from build123d import *

# Parameters (mm, degrees)
SKETCH1_W           = 190
SKETCH1_H           = 120
SKETCH1_R           = 6
SKETCH1_R_2         = 10
SKETCH1_R_3         = 2
BOSS_EXTRUDE1_DEPTH = 5


with BuildPart() as part:
    # Sketch1 → Boss-Extrude1 (new body)
    with BuildSketch(Plane.XY):
        Rectangle(SKETCH1_W, SKETCH1_H)
        with Locations((-75, 30)):
            Circle(SKETCH1_R, mode=Mode.SUBTRACT)
        with Locations((75, 30)):
            Circle(SKETCH1_R, mode=Mode.SUBTRACT)
        with Locations((75, -30)):
            Circle(SKETCH1_R, mode=Mode.SUBTRACT)
        with Locations((-75, -30)):
            Circle(SKETCH1_R, mode=Mode.SUBTRACT)
        Circle(SKETCH1_R_2, mode=Mode.SUBTRACT)
        with Locations((0, 16)):
            Circle(SKETCH1_R_3, mode=Mode.SUBTRACT)
        with Locations((13.856406461, 8)):
            Circle(SKETCH1_R_3, mode=Mode.SUBTRACT)
        with Locations((13.856406461, -8)):
            Circle(SKETCH1_R_3, mode=Mode.SUBTRACT)
        with Locations((0, -16)):
            Circle(SKETCH1_R_3, mode=Mode.SUBTRACT)
        with Locations((-13.856406461, -8)):
            Circle(SKETCH1_R_3, mode=Mode.SUBTRACT)
        with Locations((-13.856406461, 8)):
            Circle(SKETCH1_R_3, mode=Mode.SUBTRACT)
    extrude(amount=BOSS_EXTRUDE1_DEPTH)


solid = part.part
Design review of the part built by this model. Coordinates are the model's own, in mm. Round coordinates to 2 decimals unless told otherwise and drop trailing zeros. Order: outer loops, then holes, each group sorted by start corner. A loop starts at its lowest first (then second) coordinate and runs counter-clockwise, first axis right, second up.
1) For L1, parallel to Y at x = -75, z = 3.2; L2, parallel to Y at x = -13, z = 1.75; L3, parallel to X at y = -16.5, z = 3.2, list the stretches that pass through material, from the lowest coordinate up.
The answers:
L1: y = -60 to -36, -24 to 24, 36 to 60
L2: y = -60 to -9.81, -6.19 to 6.19, 9.81 to 60
L3: x = -95 to -1.94, 1.94 to 95
2) Consider section D-D (z = 2.7). Count the separate pieces of the cut face and the enclosed holes in it, plus the area to 3 significant figures.
The answers:
separate pieces: 1
enclosed holes: 11
area: 22,000 mm2
3) Clearance check with a flat-ended pin moving along its axis: pin 1 Ø6.5 at (x, y) = (0, -16) entering from +Z. State where the tip first meets the part, or that it passes through.
The answers:
pin 1: stops at z = 5
4) Consider section A-A (x = 0). State the section outline as (y, z) points.
The answers:
outline: (-60, 0) - (-18, 0) - (-18, 5) - (-60, 5) - close; (-14, 0) - (-10, 0) - (-10, 5) - (-14, 5) - close; (10, 0) - (14, 0) - (14, 5) - (10, 5) - close; (18, 0) - (60, 0) - (60, 5) - (18, 5) - close
5) Consider section C-C (y = 0). State the section outline as (x, z) points.
The answers:
outline: (-95, 0) - (-10, 0) - (-10, 5) - (-95, 5) - close; (10, 0) - (95, 0) - (95, 5) - (10, 5) - close
6) Draft analysis for pull direction X (two halves, no side actions). For faces 1 (the flat face through (-1, 14, 0)), 2 (the cylindrical face through (-81, 30, 2)), 3 (the flat face through (95, -1, 2)), state which applies: released by +X, released by -X, zero draft, split by the parting line, or undercut.
The answers:
face 1: zero draft
face 2: undercut
face 3: released by +X
7) Consider section B-B (x = 75). State the section outline as (y, z) points.
The answers:
outline: (-60, 0) - (-36, 0) - (-36, 5) - (-60, 5) - close; (-24, 0) - (24, 0) - (24, 5) - (-24, 5) - close; (36, 0) - (60, 0) - (60, 5) - (36, 5) - close
